Part model, mm, in its own coordinate system. Face numbers are marked on the shaded views. Round coordinates to 2 decimals unless told otherwise and drop trailing zeros. Write each loop counter-clockwise with the first axis right and the second up, starting at its lowest first coordinate (ties: lowest second). Pieces come first, ordered by that corner, then holes. Notation, with made-up numbers: (86, 80) -> (119, 80) arc R9 ccw to (119, 96) -> close; hole circle Ø4 at (29.25, -14.5). An arc over 180 degrees is marked (long way). Return JSON: item names as keys, results as strings. Group by question number.
(1) Mould opens along Y. For the marked faces 1, 2 and 3 say: +Y half, -Y half, draft (parallel to the pull), parting line (faces both ways), or undercut.
(2) Saw through at D-D (z = -53.5). List the corners of the cut face in (x, y).
(3) Saw through at C-C (z = 27). List the corners of the cut face in (x, y), plus the area to 3 significant figures.
(4) Drop flat-ended pins along their axis: pin 1 Ø6 at (x, z) = (20.5, 29) entering from -Y; pin 2 Ø1.5 at (x, z) = (-27.5, 15.5) entering from -Y; pin 3 Ø3 at (x, z) = (-33, -17) entering from -Y. Give the stop position or say it passes through.
(5) Drill centre lines: L1, parallel to Z at x = 16.5, y = 10; L2, parallel to Y at x = -4, z = -49; L3, parallel to Y at x = 1, z = -48. Where is each one in solid material? Low to high. Write a range as from..to.
from build123d import *

# Parameters (mm, degrees)
F0_R     = 44.45
F1_DEPTH = 63.5
F3_T     = -2.54
F4_R     = 1.26999
F5_R     = 30.988
F6_DEPTH = 25.4


# Not quite as in the source:
# - a fillet or chamfer that OpenCascade refuses, or shapes differently, is made with other operations: its cross-section is extruded or revolved along the edge and cut away or added
# - a fillet or chamfer is up to 0.001 mm smaller than in the source, because OpenCascade refuses the exact size


with BuildPart() as f1:
    # F0 (on Top) → F1 (new body, symmetric)
    with BuildSketch(Plane.XY):
        Circle(F0_R)
    extrude(amount=F1_DEPTH, both=True)

    # F2: chamfer of 152.4 x 13.3332723214 on 1 edges, made by hand

    # F2_s1 → F2_t2 (revolve, cut)
    with BuildSketch(Plane.XZ):
        Polygon((44.45, 88.9), (31.1167276786, -63.5), (44.45, -63.5), align=None)
    revolve(axis=Axis((0, 0, -63.5), (0, 0, 1)), mode=Mode.SUBTRACT)

    # F3
    f3_openings = [f1.faces().sort_by_distance(p)[0] for p in [
        (0, 0, 63.5),
    ]]
    offset(amount=F3_T, openings=f3_openings)

    # F4 (radius 1.27 in the source; OpenCascade refuses exactly that, so slightly less here)
    f4_edges = [f1.edges().sort_by_distance(p)[0] for p in [
        (-42.227788, 0, 63.5),
        (-39.678086, 0, 63.5),
    ]]
    fillet(f4_edges, radius=F4_R)

    # F5 (on face) → F6 (join)
    with BuildSketch(Plane(origin=(0, 0, -63.5), x_dir=(1, 0, 0), z_dir=(0, 0, -1))):
        Circle(F5_R)
    extrude(amount=F6_DEPTH)


solid = f1.part
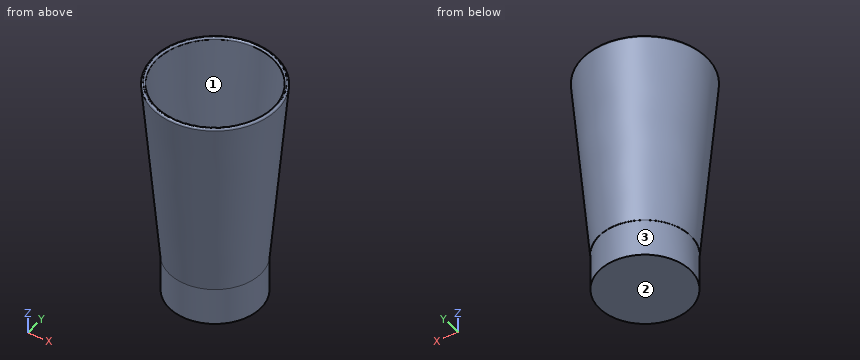
Computed values:
{
 "1": {"face 1": "undercut", "face 2": "draft", "face 3": "parting line"},
 "2": {"outline": "circle Ø63.98 at (0, 0); hole circle Ø58.88 at (0, 0)"},
 "3": {"outline": "circle Ø78.07 at (0, 0); hole circle Ø72.97 at (0, 0)", "area": "605 mm2"},
 "4": {"pin 1": "y = -35.12", "pin 2": "y = -27.04", "pin 3": "y = -15.69"},
 "5": {"L1": "-88.9..-60.96", "L2": "-32.14..-29.57, 29.57..32.14", "L3": "-32.46..-29.91, 29.91..32.46"}
}
